```python
from build123d import *

# Parameters (mm, degrees)
ESQUISSE1_W                                 = 103
ESQUISSE1_H                                 = 53
BOSS_EXTRU_1_DEPTH                          = 1.5
FRAISAGE_POUR_VIS_T_TE_FRAIS_E_M31_AT_COUNT = 2
FRAISAGE_POUR_VIS_T_TE_FRAIS_E_M31_AT_PITCH = 95.02
FRAISAGE_POUR_VIS_T_TE_FRAIS_E_M31_2_COUNT  = 2
FRAISAGE_POUR_VIS_T_TE_FRAIS_E_M31_2_PITCH  = 105.137055314
FRAISAGE_POUR_VIS_T_TE_FRAIS_E_M31_3_COUNT  = 2
FRAISAGE_POUR_VIS_T_TE_FRAIS_E_M31_3_PITCH  = 45
CONG_1_R                                    = 3.99
ESQUISSE5_R                                 = 6.5
ENL_V_MAT_EXTRU_1_DEPTH                     = 2.5


with BuildPart() as part:
    # Esquisse1 → Boss.-Extru.1 (new body)
    with BuildSketch(Plane(origin=(0, 0, -0.75), x_dir=(-1, 0, 0), z_dir=(0, 0, -1))):
        Rectangle(ESQUISSE1_W, ESQUISSE1_H)
    extrude(amount=-BOSS_EXTRU_1_DEPTH)

    # Esquisse2 → Fraisage pour vis à tête fraisée M31 (revolve, cut)
    with BuildSketch(Plane(origin=(-47.51, 22.5, 0.75), x_dir=(0, -1, 0), z_dir=(1, 0, 0))):
        Polygon((0, 0), (0, 1.5), (1.75, 1.5), (1.75, 1.125), (2.875, 0), align=None)
    fraisage_pour_vis_t_te_frais_e_m31 = revolve(axis=Axis((-47.51, 22.5, 7.1), (0, 0, -1)), mode=Mode.SUBTRACT)

    # Fraisage pour vis à tête fraisée M31 at: Fraisage pour vis à tête fraisée M31 ×2
    with Locations(*[(i * FRAISAGE_POUR_VIS_T_TE_FRAIS_E_M31_AT_PITCH, 0, 0) for i in range(1, FRAISAGE_POUR_VIS_T_TE_FRAIS_E_M31_AT_COUNT)]):
        add(fraisage_pour_vis_t_te_frais_e_m31, mode=Mode.SUBTRACT)

    # Fraisage pour vis _ t_te frais_e M31 2: Fraisage pour vis à tête fraisée M31 ×2
    with Locations(*[Vector(0.903772697, -0.428012748, 0) * (i * FRAISAGE_POUR_VIS_T_TE_FRAIS_E_M31_2_PITCH) for i in range(1, FRAISAGE_POUR_VIS_T_TE_FRAIS_E_M31_2_COUNT)]):
        add(fraisage_pour_vis_t_te_frais_e_m31, mode=Mode.SUBTRACT)

    # Fraisage pour vis _ t_te frais_e M31 3: Fraisage pour vis à tête fraisée M31 ×2
    with Locations(*[(0, -i * FRAISAGE_POUR_VIS_T_TE_FRAIS_E_M31_3_PITCH, 0) for i in range(1, FRAISAGE_POUR_VIS_T_TE_FRAIS_E_M31_3_COUNT)]):
        add(fraisage_pour_vis_t_te_frais_e_m31, mode=Mode.SUBTRACT)

    # Congé1
    cong_1_edges = [part.edges().sort_by_distance(p)[0] for p in [
        (51.5, 26.5, 0),
        (-51.5, 26.5, 0),
        (-51.5, -26.5, 0),
        (51.5, -26.5, 0),
    ]]
    fillet(cong_1_edges, radius=CONG_1_R)

    # Esquisse5 → Enlèv. mat.-Extru.1 (cut, through all)
    with BuildSketch(Plane.XY.offset(0.75)):
        with Locations((-7.5, -8)):
            Circle(ESQUISSE5_R)
        with BuildLine():
            Line((-28.5, -17.6), (-38.5, -17.6))
            ThreePointArc((-38.5, -17.6), (-39.560660172, -17.160660172), (-40, -16.1))
            Line((-40, -16.1), (-40, 0.1))
            ThreePointArc((-40, 0.1), (-39.560660172, 1.160660172), (-38.5, 1.6))
            Line((-38.5, 1.6), (-28.5, 1.6))
            ThreePointArc((-28.5, 1.6), (-27.439339828, 1.160660172), (-27, 0.1))
            Line((-27, 0.1), (-27, -16.1))
            ThreePointArc((-27, -16.1), (-27.439339828, -17.160660172), (-28.5, -17.6))
        make_face()
        with BuildLine():
            Line((31.16, 4), (12.16, 4))
            ThreePointArc((12.16, 4), (11.099339828, 4.439339828), (10.66, 5.5))
            Line((10.66, 5.5), (10.66, 8))
            Line((10.66, 8), (9.16, 8))
            ThreePointArc((9.16, 8), (7.66, 9.5), (9.16, 11))
            Line((9.16, 11), (10.66, 11))
            Line((10.66, 11), (10.66, 13.5))
            ThreePointArc((10.66, 13.5), (11.099339828, 14.560660172), (12.16, 15))
            Line((12.16, 15), (31.16, 15))
            ThreePointArc((31.16, 15), (32.220660172, 14.560660172), (32.66, 13.5))
            Line((32.66, 13.5), (32.66, 11))
            Line((32.66, 11), (34.16, 11))
            ThreePointArc((34.16, 11), (35.66, 9.5), (34.16, 8))
            Line((34.16, 8), (32.66, 8))
            Line((32.66, 8), (32.66, 5.5))
            ThreePointArc((32.66, 5.5), (32.220660172, 4.439339828), (31.16, 4))
        make_face()
        with BuildLine():
            Line((-13.45, 4.35), (-1.55, 4.35))
            ThreePointArc((-1.55, 4.35), (-1.019669914, 4.569669914), (-0.8, 5.1))
            Line((-0.8, 5.1), (-0.8, 15.25))
            ThreePointArc((-0.8, 15.25), (-1.019669914, 15.780330086), (-1.55, 16))
            Line((-1.55, 16), (-13.45, 16))
            ThreePointArc((-13.45, 16), (-13.980330086, 15.780330086), (-14.2, 15.25))
            Line((-14.2, 15.25), (-14.2, 5.1))
            ThreePointArc((-14.2, 5.1), (-13.980330086, 4.569669914), (-13.45, 4.35))
        make_face()
    extrude(amount=-ENL_V_MAT_EXTRU_1_DEPTH, mode=Mode.SUBTRACT)


solid = part.part
```
Design review of the part built by this model. Coordinates are the model's own, in mm. Coordinates: 2 decimals unless noted, no trailing zeros. Loops run counter-clockwise (first coordinate to the right, second up) from the corner with the lowest first, then second, coordinate; pieces in that order, holes last. Notation, with made-up numbers: (46, 79) -> (76, 79) arc R26 ccw to (76, 103) -> close; hole circle Ø8 at (24, 55). An arc over 180 degrees is marked (long way). Answer as a JSON object with one key per item and string values.
Q1. Clearance check with flat-ended pins moving along their axes: pin 1 Ø4.5 at (x, y) = (-47.51, 22.5) entering from +Z (3 decimals); pin 2 Ø5.5 at (x, y) = (-47.51, -22.5) entering from +Z (3 decimals); pin 3 Ø10.5 at (x, y) = (-7.5, -8) entering from +Z. State where each tip first meets the part, or that it passes through.
Answer block:
{"pin 1": "stops at z = 0.125", "pin 2": "stops at z = 0.625", "pin 3": "passes through"}
Q2. Take a section at A-A on x = -7.5. Give the boundary of the cut face in (y, z).
Answer block:
{"outline": "(-26.5, -0.75) -> (-14.5, -0.75) -> (-14.5, 0.75) -> (-26.5, 0.75) -> close; (-1.5, -0.75) -> (4.35, -0.75) -> (4.35, 0.75) -> (-1.5, 0.75) -> close; (16, -0.75) -> (26.5, -0.75) -> (26.5, 0.75) -> (16, 0.75) -> close"}
Q3. Take a section at C-C on z = 0.05. Give the number of separate pieces and of enclosed holes in the cut face, plus the area to 3 significant figures.
Answer block:
{"separate pieces": "1", "enclosed holes": "8", "area": "4,590 mm^2"}
Q4. The part is to be moulded in two halves that separate along Y. For faces 1 (the cylindrical face through (-50.3, 25.36, 0.01)), 2 (the flat face through (1, 0, -0.75)), 3 (the cylindrical face through (-1.5, -10.5, 0)), say which applies: +Y half, -Y half, draft (parallel to the pull), parting line (faces both ways), or undercut.
Answer block:
{"face 1": "+Y half", "face 2": "draft", "face 3": "undercut"}
Q5. Take a section at B-B on y = 9.5. Give the boundary of the cut face in (x, z).
Answer block:
{"outline": "(-51.5, -0.75) -> (-14.2, -0.75) -> (-14.2, 0.75) -> (-51.5, 0.75) -> close; (-0.8, -0.75) -> (7.66, -0.75) -> (7.66, 0.75) -> (-0.8, 0.75) -> close; (35.66, -0.75) -> (51.5, -0.75) -> (51.5, 0.75) -> (35.66, 0.75) -> close"}
Q6. To check wall thickness, follow L1, parallel to Y at x = -47.51, z = -0.5; L2, parallel to X at y = 22.5, z = -0.55; L3, parallel to Y at x = -7.5, z = 0.3. State the ranges of each line that lie inside material, in increasing order.
Answer block:
{"L1": "y = -26.5 to -24.25, -20.75 to 20.75, 24.25 to 26.5", "L2": "x = -51.5 to -49.26, -45.76 to 45.76, 49.26 to 51.5", "L3": "y = -26.5 to -14.5, -1.5 to 4.35, 16 to 26.5"}
